```python
from build123d import *

# Parameters (mm, degrees)
BOSS_EXTRUDE1_DEPTH = 6.2
CUT_EXTRUDE1_DEPTH  = 1


with BuildPart() as part:
    # Sketch1 → Boss-Extrude1 (new body)
    with BuildSketch(Plane(origin=(0, 0, 0), x_dir=(1, 0, 0), z_dir=(0, 1, 0))):
        Polygon((0, 0), (91.95, 0), (98.15, 0), (98.15, 3), (93.712314791, 3), (91.95, 3), (91.95, 7), (93.712314791, 7), (98.15, 7), (98.15, 10), (91.95, 10), (0, 10), align=None)
    extrude(amount=BOSS_EXTRUDE1_DEPTH)

    # Sketch2 → Cut-Extrude1 (cut)
    with BuildSketch(Plane(origin=(0, 6.2, 0), x_dir=(1, 0, 0), z_dir=(0, 1, 0))):
        with BuildLine():
            Line((11.210257143, 3.497319833), (10.982562832, 3.655688223))
            Line((10.982562832, 3.655688223), (11.8653553, 4.94616799))
            add(Edge.make_bspline(
                [(11.8653553, 4.94616799), (11.809030133, 4.939279997), (11.698122738, 4.925717154), (11.586419796, 4.923225546), (11.531446045, 4.92199932)],
                knots=[0, 0, 0, 0, 0.000170115, 0.000334967, 0.000334967, 0.000334967, 0.000334967], degree=3))
            add(Edge.make_bspline(
                [(11.531446045, 4.92199932), (11.498115759, 4.922853011), (11.432691322, 4.924528731), (11.336505466, 4.937810943), (11.244080707, 4.958267131), (11.155662077, 4.988791358), (11.070917241, 5.026726448), (10.990031201, 5.073768168), (10.913112843, 5.129109589), (10.840988264, 5.192458089), (10.775391186, 5.262016036), (10.716950052, 5.335635798), (10.668380597, 5.414172571), (10.62803398, 5.496024271), (10.59743564, 5.582367353), (10.575153909, 5.672219309), (10.561435774, 5.76620987), (10.559803737, 5.830186239), (10.558975092, 5.862669392)],
                knots=[0, 0, 0, 0, 9.9954e-05, 0.000196201, 0.000290782, 0.000383503, 0.000476303, 0.000568919, 0.000663705, 0.000760153, 0.000856434, 0.000950205, 0.001041624, 0.001132931, 0.001223461, 0.001315861, 0.001410305, 0.001507717, 0.001507717, 0.001507717, 0.001507717], degree=3))
            add(Edge.make_bspline(
                [(10.558975092, 5.862669392), (10.560548472, 5.907090956), (10.563636698, 5.994281474), (10.588491067, 6.121674964), (10.629367232, 6.242131329), (10.686361545, 6.355333862), (10.758148043, 6.459654147), (10.844425121, 6.553641957), (10.944668003, 6.635960503), (11.05659312, 6.706721344), (11.17756336, 6.763630949), (11.304262786, 6.8055766), (11.435720595, 6.83024975), (11.524772696, 6.833502638), (11.569607103, 6.835140346)],
                knots=[0, 0, 0, 0, 0.000133185, 0.000261414, 0.000387724, 0.00051373, 0.000640399, 0.00076644, 0.000895188, 0.001028407, 0.001162697, 0.001295241, 0.001427846, 0.0015623, 0.0015623, 0.0015623, 0.0015623], degree=3))
            add(Edge.make_bspline(
                [(11.569607103, 6.835140346), (11.613593027, 6.833480127), (11.700505066, 6.83019969), (11.828311522, 6.806174946), (11.950722301, 6.765683107), (12.067058825, 6.709726396), (12.174772434, 6.639585287), (12.271633349, 6.556006112), (12.355431159, 6.458936812), (12.426028537, 6.35072511), (12.482697788, 6.234459349), (12.523584787, 6.113098219), (12.548754046, 5.987514522), (12.551925714, 5.902429535), (12.553526374, 5.859489304)],
                knots=[0, 0, 0, 0, 0.000131915, 0.000260652, 0.000388569, 0.000517718, 0.000646848, 0.000773094, 0.000900237, 0.001030248, 0.001159674, 0.001287189, 0.001413545, 0.001542287, 0.001542287, 0.001542287, 0.001542287], degree=3))
            add(Edge.make_bspline(
                [(12.553526374, 5.859489304), (12.552457389, 5.826157458), (12.55028922, 5.758552146), (12.535106998, 5.65583605), (12.50932583, 5.551105292), (12.480068932, 5.462457844), (12.451827608, 5.38924375), (12.425247296, 5.33141196), (12.395754128, 5.270541528), (12.361356391, 5.207270729), (12.324379165, 5.140793001), (12.282596821, 5.071775108), (12.236962481, 5.000124436), (12.204459807, 4.95182172), (12.187816238, 4.927087461)],
                knots=[0, 0, 0, 0, 9.9984e-05, 0.000202793, 0.000310776, 0.000423207, 0.000482616, 0.000546097, 0.000614079, 0.0006855, 0.000762103, 0.000842274, 0.000927493, 0.001016928, 0.001016928, 0.001016928, 0.001016928], degree=3))
            Line((12.187816238, 4.927087461), (11.210257143, 3.497319833))
        make_face()
        with BuildLine():
            add(Edge.make_bspline(
                [(11.584235509, 5.247640346), (11.609484936, 5.248330123), (11.658636986, 5.249672883), (11.730643536, 5.257845553), (11.798610492, 5.27233624), (11.862719411, 5.293127693), (11.923613101, 5.318216243), (11.980324341, 5.350158545), (12.032900595, 5.388273635), (12.081693929, 5.431099863), (12.1250227, 5.478680036), (12.163615307, 5.528479554), (12.196418107, 5.580717021), (12.22232908, 5.636046624), (12.243632945, 5.69312152), (12.258344999, 5.752860828), (12.266495072, 5.814953306), (12.26788443, 5.857134231), (12.268590477, 5.878569833)],
                knots=[0, 0, 0, 0, 7.5753e-05, 0.000147465, 0.000217073, 0.000283852, 0.000349411, 0.000414338, 0.000478589, 0.000543925, 0.000608743, 0.000671332, 0.000732749, 0.000793345, 0.000854313, 0.000915245, 0.00097749, 0.001041807, 0.001041807, 0.001041807, 0.001041807], degree=3))
            add(Edge.make_bspline(
                [(12.268590477, 5.878569833), (12.267982991, 5.900014387), (12.266785866, 5.94227351), (12.257181673, 6.004457916), (12.240285935, 6.064051089), (12.217615995, 6.121379279), (12.187752636, 6.175971473), (12.151917331, 6.228513071), (12.109342895, 6.27867093), (12.060354853, 6.325265401), (12.007527794, 6.368216709), (11.951230054, 6.40612265), (11.891925666, 6.437891878), (11.829976436, 6.464107372), (11.765253291, 6.484565054), (11.69779453, 6.499276521), (11.62725927, 6.507415184), (11.579379103, 6.50879576), (11.554978698, 6.50949932)],
                knots=[0, 0, 0, 0, 6.4316e-05, 0.000126743, 0.000188161, 0.000249812, 0.000311283, 0.000374438, 0.00044032, 0.000508243, 0.00057698, 0.000644365, 0.000711521, 0.0007785, 0.000845884, 0.000914871, 0.00098532, 0.001058531, 0.001058531, 0.001058531, 0.001058531], degree=3))
            add(Edge.make_bspline(
                [(11.554978698, 6.50949932), (11.530790501, 6.508794623), (11.48333346, 6.507412013), (11.413425258, 6.499291991), (11.346422627, 6.484466116), (11.281887014, 6.464116848), (11.219939625, 6.437889922), (11.160638034, 6.406120985), (11.104327126, 6.368225435), (11.051550715, 6.325231606), (11.002476171, 6.278887812), (10.960633727, 6.228293345), (10.924716411, 6.175998805), (10.894894087, 6.121372015), (10.872213232, 6.064053027), (10.855320416, 6.004457391), (10.845715438, 5.942273646), (10.84451842, 5.900014433), (10.843910989, 5.878569833)],
                knots=[0, 0, 0, 0, 7.2576e-05, 0.000142393, 0.000210758, 0.000278143, 0.000345121, 0.000412278, 0.000479663, 0.0005484, 0.000616323, 0.000681795, 0.00074495, 0.000806421, 0.000868072, 0.00092949, 0.000991917, 0.001056233, 0.001056233, 0.001056233, 0.001056233], degree=3))
            add(Edge.make_bspline(
                [(10.843910989, 5.878569833), (10.844460651, 5.857117539), (10.845544684, 5.814809687), (10.856002036, 5.752646459), (10.87349019, 5.693057883), (10.896912066, 5.635464556), (10.927756365, 5.580426514), (10.965605856, 5.528204693), (11.009970173, 5.478207106), (11.060256265, 5.431210563), (11.115290954, 5.388073947), (11.174070859, 5.350399958), (11.235584069, 5.31858424), (11.300047119, 5.293055985), (11.366982288, 5.272543976), (11.436991157, 5.25787226), (11.509842201, 5.249751275), (11.559199827, 5.24835074), (11.584235509, 5.247640346)],
                knots=[0, 0, 0, 0, 6.4316e-05, 0.000126844, 0.000188436, 0.000250326, 0.000312966, 0.000377217, 0.000443451, 0.000513196, 0.000583426, 0.000652939, 0.000722346, 0.000790847, 0.000860662, 0.000932137, 0.001005113, 0.00108023, 0.00108023, 0.00108023, 0.00108023], degree=3))
        make_face(mode=Mode.SUBTRACT)
        Polygon((13.164103297, 6.75373009), (15.117949451, 6.75373009), (13.449039195, 3.497319833), (13.202900372, 3.632791588), (14.635848089, 6.428089064), (13.164103297, 6.428089064), align=None)
    extrude(amount=-CUT_EXTRUDE1_DEPTH, mode=Mode.SUBTRACT)


solid = part.part
```
Can you work these out from the model? Positions are in its coordinate system, mm. A direction names the side the tool comes from. Give positions to 0.01 mm unless a question says otherwise; leave off trailing zeros. Order: outer loops, then holes, each group sorted by start corner. A loop starts at its lowest first (then second) coordinate and runs counter-clockwise, first axis right, second up. Notation, with made-up numbers: M 45,2 L 70,2 A18 cw 70,14 Z; hole C -28.75,-21 d2. An arc over 180 degrees is marked long. Write item = value, one per line. Start each with the question number.
Q1. Will these pins go through, and if not, where does the flat tip stop? pin 1 Ø0.8 at (x, y) = (14, 6) entering from +Z; pin 2 Ø3 at (y, z) = (2, -5) entering from +X.
Q2. For faces 4 (the flat face through (98.15, 3, -1)), 5 (the flat face through (11.7, 5.2, -5.1)), 6 (the flat face through (95, 3, -3)), which set-ups out of +Z, -Z, +X, -X, +Y, -Y let a thin tool reach every point of the face, with its end or its side?
Q3. Suppose I cut it at A-A (y = 1.25). Write out the boundary of the cut face in (x, z).
Q4. We'd pull the mould along X, two halves only. Please class faces 1 (the flat face through (14.295, 5.707, -5.148)), 2 (the flat face through (91.95, 3, -5)), 3 (the flat face through (95, 3, -7)): pulls with the +X half, pulls with the -X half, needs draft (parallel to the pull), parting line crosses it, or undercut.
Q5. I need wall thicknesses on probe 1 along Z at (x, y) = (94, 3); probe 2 along X at (y, z) = (0.5, -4.25). Which ranges of each line are inside material? Lowest first, please. Write a range as [from, to].
Check result:
q1.pin_1 = 0
q1.pin_2 = 91.95
q2.face_4 = +Z, -Z, +X, +Y, -Y
q2.face_5 = +Y
q2.face_6 = +X, +Y, -Y
q3.outline = M 0,-10 L 98.15,-10 L 98.15,-7 L 91.95,-7 L 91.95,-3 L 98.15,-3 L 98.15,0 L 0,0 Z
q4.face_1 = undercut
q4.face_2 = pulls with the +X half
q4.face_3 = needs draft
q5.probe_1 = [-10, -7], [-3, 0]
q5.probe_2 = [0, 91.95]
